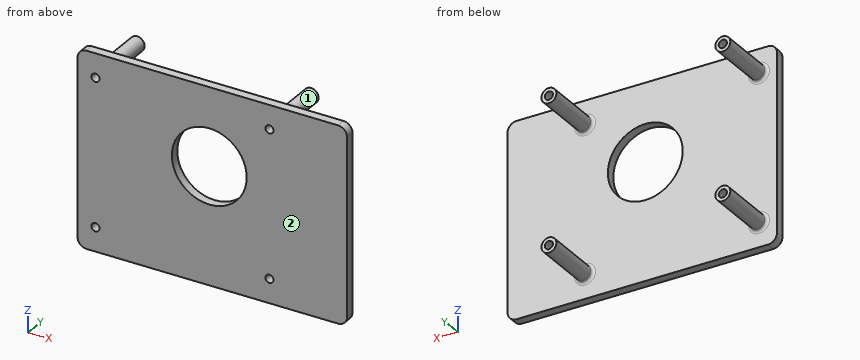
from build123d import *

# Parameters (mm, degrees)
SKIZZE1_W                       = 90
SKIZZE1_H                       = 65
AUFSATZ_LINEAR_AUSTRAGEN1_DEPTH = 3
SKIZZE3_R                       = 2.5
AUFSATZ_LINEAR_AUSTRAGEN2_DEPTH = 20
SKIZZE4_R                       = 1.364499713
SCHNITT_LINEAR_AUSTRAGEN2_DEPTH = 61.085355953
VERRUNDUNG1_R                   = 3
VERRUNDUNG2_R                   = 1
SKIZZE5_R                       = 12.500347999
SCHNITT_LINEAR_AUSTRAGEN3_DEPTH = 61.085355953


with BuildPart() as part:
    # Skizze1 → Aufsatz-Linear austragen1 (new body)
    with BuildSketch(Plane(origin=(0, 0, 0), x_dir=(1, 0, 0), z_dir=(0, 1, 0))):
        Rectangle(SKIZZE1_W, SKIZZE1_H)
    extrude(amount=AUFSATZ_LINEAR_AUSTRAGEN1_DEPTH)

    # Skizze3 → Aufsatz-Linear austragen2 (add)
    with BuildSketch(Plane(origin=(0, 3, 0), x_dir=(1, 0, 0), z_dir=(0, 1, 0))):
        with Locations(Location((-39, 24.5, 0), (0, 0, 270))):
            Circle(SKIZZE3_R)
        with Locations(Location((19.085512482, 24.5, 0), (0, 0, 270))):
            Circle(SKIZZE3_R)
        with Locations(Location((19.085512482, -24.5, 0), (0, 0, 270))):
            Circle(SKIZZE3_R)
        with Locations(Location((-39, -24.5, 0), (0, 0, 270))):
            Circle(SKIZZE3_R)
    extrude(amount=AUFSATZ_LINEAR_AUSTRAGEN2_DEPTH)

    # Skizze4 → Schnitt-Linear austragen2 (cut, through all)
    with BuildSketch(Plane(origin=(0, 23, 0), x_dir=(1, 0, 0), z_dir=(0, 1, 0))):
        with Locations(Location((19.085512482, 24.5, 0), (0, 0, 270))):
            Circle(SKIZZE4_R)
        with Locations(Location((-39, 24.5, 0), (0, 0, 270))):
            Circle(SKIZZE4_R)
        with Locations(Location((-39, -24.5, 0), (0, 0, 270))):
            Circle(SKIZZE4_R)
        with Locations(Location((19.085512482, -24.5, 0), (0, 0, 270))):
            Circle(SKIZZE4_R)
    extrude(amount=-SCHNITT_LINEAR_AUSTRAGEN2_DEPTH, mode=Mode.SUBTRACT)

    # Verrundung1
    verrundung1_edges = [part.edges().sort_by_distance(p)[0] for p in [
        (-45, 1.5, 32.5),
        (-45, 1.5, -32.5),
        (45, 1.5, -32.5),
        (45, 1.5, 32.5),
    ]]
    fillet(verrundung1_edges, radius=VERRUNDUNG1_R)

    # Verrundung2
    verrundung2_edges = [part.edges().sort_by_distance(p)[0] for p in [
        (-39, 3, -27),
        (19.085512482, 3, -27),
        (19.085512482, 3, 22),
        (-39, 3, 22),
    ]]
    fillet(verrundung2_edges, radius=VERRUNDUNG2_R)

    # Skizze5 → Schnitt-Linear austragen3 (cut, through all)
    with BuildSketch(Plane.XZ):
        with Locations(Location((-1, 6.5, 0), (0, 0, 270))):
            Circle(SKIZZE5_R)
    extrude(amount=-SCHNITT_LINEAR_AUSTRAGEN3_DEPTH, mode=Mode.SUBTRACT)


solid = part.part
The listing builds one solid part. Answer for the finished solid, in the listing's coordinates (mm). Face numbers are marked on the shaded views. Give positions to 0.01 mm unless a question says otherwise; leave off trailing zeros. Write each loop counter-clockwise with the first axis right and the second up, starting at its lowest first coordinate (ties: lowest second). Pieces come first, ordered by that corner, then holes.
Item 1: Section D-D, the plane x = -39 is taken. Write down the section's boundary in (y, z), plus the area to 3 significant figures.
Item 2: Flat-ended cylindrical pins translate along their axes: P1, Ø6, axis at y = 19, z = 20.5, coming from the -X side; P2, Ø4.5, axis at x = -39, z = -24.5, coming from the +Y side. Find the tip coordinate at first contact, or state that the pin passes through.
Item 3: Find the intervals of material crossed by line 1 along X through (y, z) = (6.75, -24.5); line 2 along Z through (x, y) = (17, 12); line 3 along Y through (x, z) = (-31, 5.5), in increasing order.
Item 4: Section A-A, the plane z = 6.5 is taken. Write down the section's boundary in (x, y), plus the area to 3 significant figures.
Item 5: Section B-B, the plane x = -1 is taken. Write down the section's boundary in (y, z).
Item 6: Section C-C, the plane y = 9 is taken. Write down the section's boundary in (x, z).
Item 7: Determine the mould class of the marked faces 1 and 2 for opening direction Z: released by +Z, released by -Z, zero draft, split by the parting line, or undercut.
Completed:
1. outline: (0, -32.5) - (3, -32.5) - (3, -28) arc R1 cw to (4, -27) - (23, -27) - (23, -25.86) - (0, -25.86) - close; (0, -23.14) - (23, -23.14) - (23, -22) - (4, -22) arc R1 cw to (3, -21) - (3, 21) arc R1 cw to (4, 22) - (23, 22) - (23, 23.14) - (0, 23.14) - close; (0, 25.86) - (23, 25.86) - (23, 27) - (4, 27) arc R1 cw to (3, 28) - (3, 32.5) - (0, 32.5) - close
1. area: 270 mm2
2. P1: stops at x = -41.29
2. P2: stops at y = 23
3. line 1: x = -41.5 to -40.36, -37.64 to -36.5, 16.59 to 17.72, 20.45 to 21.59
3. line 2: z = -25.88 to -23.12, 23.12 to 25.88
3. line 3: y = 0 to 3
4. outline: (-45, 0) - (-13.5, 0) - (-13.5, 3) - (-45, 3) - close; (11.5, 0) - (45, 0) - (45, 3) - (11.5, 3) - close
4. area: 195 mm2
5. outline: (0, -32.5) - (3, -32.5) - (3, -6) - (0, -6) - close; (0, 19) - (3, 19) - (3, 32.5) - (0, 32.5) - close
6. outline: circle Ø5 at (-39, -24.5); circle Ø5 at (-39, 24.5); circle Ø5 at (19.09, -24.5); circle Ø5 at (19.09, 24.5); hole circle Ø2.73 at (-39, -24.5); hole circle Ø2.73 at (-39, 24.5); hole circle Ø2.73 at (19.09, -24.5); hole circle Ø2.73 at (19.09, 24.5)
7. face 1: undercut
7. face 2: zero draft
